```python
from build123d import *

# Parameters (mm, degrees)
SKETCH_1_R      = 1.5
SKETCH_1_W      = 5
SKETCH_1_H      = 3
EXTRUDE_1_DEPTH = 3


with BuildPart() as part:
    # 草图1 → 凸台-拉伸1 (new body)
    with BuildSketch(Plane.XY):
        with BuildLine():
            Line((0, 63.169976396), (0, 40.169976396))
            Line((0, 40.169976396), (3, 40.169976396))
            Line((3, 40.169976396), (3, 46.169976396))
            Line((3, 46.169976396), (6, 46.169976396))
            Line((6, 46.169976396), (6, 34.169976396))
            Line((6, 34.169976396), (12, 34.169976396))
            Line((12, 34.169976396), (12, 37.169976396))
            Line((12, 37.169976396), (9, 37.169976396))
            Line((9, 37.169976396), (9, 40.169976396))
            Line((9, 40.169976396), (42.5, 40.169976396))
            Line((42.5, 40.169976396), (42.5, 46.169976396))
            Line((42.5, 46.169976396), (45.5, 46.169976396))
            Line((45.5, 46.169976396), (45.5, 40.169976396))
            Line((45.5, 40.169976396), (72.5, 40.169976396))
            Line((72.5, 40.169976396), (72.5, 38.169976396))
            Line((72.5, 38.169976396), (75.5, 38.169976396))
            Line((75.5, 38.169976396), (75.5, 47.169976396))
            Line((75.5, 47.169976396), (78.5, 47.169976396))
            Line((78.5, 47.169976396), (78.5, 40.169976396))
            Line((78.5, 40.169976396), (91, 40.169976396))
            Line((91, 40.169976396), (91, 37.169976396))
            Line((91, 37.169976396), (88, 37.169976396))
            Line((88, 37.169976396), (88, 34.169976396))
            Line((88, 34.169976396), (91, 34.169976396))
            Line((91, 34.169976396), (91, 27.669976396))
            Line((91, 27.669976396), (103, 27.669976396))
            Line((103, 27.669976396), (103, 53.169976396))
            ThreePointArc((103, 53.169976396), (100.071067812, 60.241044208), (93, 63.169976396))
            Line((93, 63.169976396), (78.5, 63.169976396))
            Line((78.5, 63.169976396), (78.5, 56.169976396))
            Line((78.5, 56.169976396), (75.5, 56.169976396))
            Line((75.5, 56.169976396), (75.5, 63.169976396))
            Line((75.5, 63.169976396), (45.5, 63.169976396))
            Line((45.5, 63.169976396), (45.5, 56.169976396))
            Line((45.5, 56.169976396), (42.5, 56.169976396))
            Line((42.5, 56.169976396), (42.5, 63.169976396))
            Line((42.5, 63.169976396), (6, 63.169976396))
            Line((6, 63.169976396), (6, 56.169976396))
            Line((6, 56.169976396), (3, 56.169976396))
            Line((3, 56.169976396), (3, 63.169976396))
            Line((3, 63.169976396), (0, 63.169976396))
        make_face()
        with Locations((4.5, 51.169976396)):
            Circle(SKETCH_1_R, mode=Mode.SUBTRACT)
        with Locations((44, 51.169976396)):
            Circle(SKETCH_1_R, mode=Mode.SUBTRACT)
        with Locations((77, 51.169976396)):
            Circle(SKETCH_1_R, mode=Mode.SUBTRACT)
        with Locations((98, 30.669976396)):
            Rectangle(SKETCH_1_W, SKETCH_1_H, mode=Mode.SUBTRACT)
    extrude(amount=EXTRUDE_1_DEPTH)


solid = part.part
```
Geometry check sheet. Reference: the model listing, model coordinates, mm. A direction names the side the tool comes from. Give positions to 0.01 mm unless a question says otherwise; leave off trailing zeros. Order: outer loops, then holes, each group sorted by start corner. A loop starts at its lowest first (then second) coordinate and runs counter-clockwise, first axis right, second up.
1. Section check D-D, the plane x = 20. Enter the section's corners in (y, z).
2. Section check B-B, the plane y = 59. Enter the section's corners in (x, z).
3. Access from +Z, -Z, +X, -X, +Y, -Y to the whole of each face (thin tool, end or side, straight path). Record for faces 1 (the face through (95.5, 31, 1)), 2 (the face through (44, 56.17, 1)), 3 (the face through (6, 40, 1)).
4. Thickness scan on L1, parallel to X at y = 45, z = 2.35; L2, parallel to X at y = 40, z = 1.3; L3, parallel to Y at x = 44, z = 1.65. Record the ranges inside material, lowest first.
5. Section check C-C, the plane x = 4.5. Enter the section's corners in (y, z), and give its area (3 significant figures).
6. Gauge pin test, flat ends, axial feed: pin 1 Ø0.9 at (x, z) = (97, 1.5) entering from +Y; pin 2 Ø1.5 at (y, z) = (59.5, 1) entering from +X. Record the tip position at first contact, or that the pin passes through.
7. Release check for a two-part mould opening along X. For faces 4 (the face through (51, 50, 3)), 5 (the face through (103, 40, 1)), 6 (the face through (75.5, 43, 1)), 7 (the face through (59, 40.17, 1)) record: pulls with the +X half, pulls with the -X half, needs draft (parallel to the pull), parting line crosses it, or undercut.
8. Section check A-A, the plane x = 90. Enter the section's corners in (y, z), and give its area (3 significant figures).
Values follow:
1. outline: (40.17, 0) - (63.17, 0) - (63.17, 3) - (40.17, 3) - close
2. outline: (0, 0) - (3, 0) - (3, 3) - (0, 3) - close; (6, 0) - (42.5, 0) - (42.5, 3) - (6, 3) - close; (45.5, 0) - (75.5, 0) - (75.5, 3) - (45.5, 3) - close; (78.5, 0) - (101.12, 0) - (101.12, 3) - (78.5, 3) - close
3. face 1: +Z, -Z
3. face 2: +Z, -Z, +Y
3. face 3: +Z, -Z, -Y
4. L1: x = 0 to 3, 6 to 42.5, 45.5 to 75.5, 78.5 to 103
4. L2: x = 6 to 9, 72.5 to 75.5, 91 to 103
4. L3: y = 46.17 to 49.67, 52.67 to 56.17
5. outline: (46.17, 0) - (49.67, 0) - (49.67, 3) - (46.17, 3) - close; (52.67, 0) - (56.17, 0) - (56.17, 3) - (52.67, 3) - close
5. area: 21.0 mm2
6. pin 1: stops at y = 62.52
6. pin 2: stops at x = 101.3
7. face 4: needs draft
7. face 5: pulls with the +X half
7. face 6: undercut
7. face 7: undercut
8. outline: (34.17, 0) - (37.17, 0) - (37.17, 3) - (34.17, 3) - close; (40.17, 0) - (63.17, 0) - (63.17, 3) - (40.17, 3) - close
8. area: 78.0 mm2
